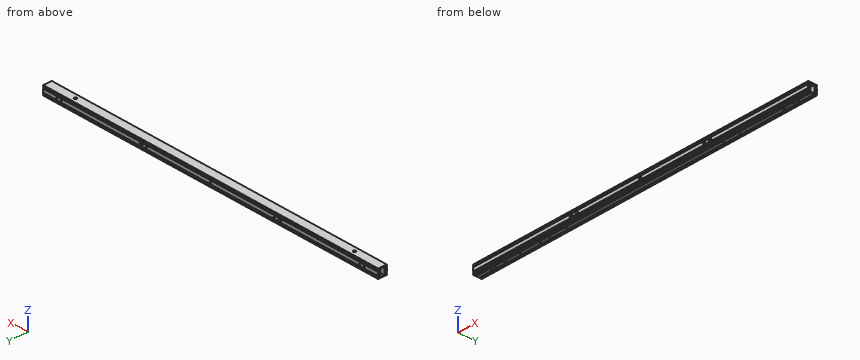
from build123d import *

# Parameters (mm, degrees)
SKETCH_1_W             = 23.5
SKETCH_1_H             = 12
EXTRUDE_1_DEPTH        = 601
HOLE_WIZARD_M6_1_D     = 5
HOLE_WIZARD_M6_1_DEPTH = 15
HOLE_WIZARD_M6_1_TIP   = 1.502151548
HOLE_WIZARD_M6_2_D     = 5
HOLE_WIZARD_M6_2_DEPTH = 15
HOLE_WIZARD_M6_2_TIP   = 1.502151548
SKETCH_8_R             = 4.5
CUT_EXTRUDE_1_DEPTH    = 602.935212461
HOLE_WIZARD_M6_3_D     = 5
HOLE_WIZARD_M6_3_DEPTH = 15
HOLE_WIZARD_M6_3_TIP   = 1.502151548
SKETCH_10_R            = 5.05
CUT_EXTRUDE_15_DEPTH   = 602.935212461
SKETCH_13_R            = 4.5
CUT_EXTRUDE_16_DEPTH   = 15
HOLE_WIZARD_M6_4_D     = 5
HOLE_WIZARD_M6_4_DEPTH = 15
HOLE_WIZARD_M6_4_TIP   = 1.502151548
HOLE_WIZARD_M6_5_D     = 5
HOLE_WIZARD_M6_5_DEPTH = 15
HOLE_WIZARD_M6_5_TIP   = 1.502151548


with BuildPart() as part:
    # 草图1 → 凸台-拉伸1 (new, symmetric)
    with BuildSketch(Plane(origin=(0, 0, 0), x_dir=(0, 0, -1), z_dir=(1, 0, 0))):
        with BuildLine():
            Line((-14, 15), (-11.5, 15))
            Line((-11.5, 15), (-11.5, 13.5))
            Line((-11.5, 13.5), (-11.4, 13.5))
            ThreePointArc((-11.4, 13.5), (-11.117157288, 13.382842712), (-11, 13.1))
            Line((-11, 13.1), (-11, 12))
            Line((-11, 12), (-9.5, 12))
            Line((-9.5, 12), (-9.5, 15))
            Line((-9.5, 15), (-8, 15))
            Line((-8, 15), (-8, 12.5))
            Line((-8, 12.5), (-5, 12.5))
            Line((-5, 12.5), (-5, 15))
            Line((-5, 15), (5, 15))
            Line((5, 15), (5, 12.5))
            Line((5, 12.5), (8, 12.5))
            Line((8, 12.5), (8, 15))
            Line((8, 15), (9.5, 15))
            Line((9.5, 15), (9.5, 12))
            Line((9.5, 12), (11, 12))
            Line((11, 12), (11, 13.1))
            ThreePointArc((11, 13.1), (11.117157288, 13.382842712), (11.4, 13.5))
            Line((11.4, 13.5), (11.5, 13.5))
            Line((11.5, 13.5), (11.5, 15))
            Line((11.5, 15), (14, 15))
            ThreePointArc((14, 15), (14.707106781, 14.707106781), (15, 14))
            Line((15, 14), (15, 8))
            Line((15, 8), (12.5, 8))
            Line((12.5, 8), (12.5, 5))
            Line((12.5, 5), (15, 5))
            Line((15, 5), (15, -5))
            Line((15, -5), (12.5, -5))
            Line((12.5, -5), (12.5, -8))
            Line((12.5, -8), (15, -8))
            Line((15, -8), (15, -14))
            ThreePointArc((15, -14), (14.707106781, -14.707106781), (14, -15))
            Line((14, -15), (11.5, -15))
            Line((11.5, -15), (11.5, -13.5))
            Line((11.5, -13.5), (11.4, -13.5))
            ThreePointArc((11.4, -13.5), (11.117157288, -13.382842712), (11, -13.1))
            Line((11, -13.1), (11, -12))
            Line((11, -12), (9.5, -12))
            Line((9.5, -12), (9.5, -15))
            Line((9.5, -15), (8, -15))
            Line((8, -15), (8, -12.5))
            Line((8, -12.5), (5, -12.5))
            Line((5, -12.5), (5, -15))
            Line((5, -15), (-5, -15))
            Line((-5, -15), (-5, -12.5))
            Line((-5, -12.5), (-8, -12.5))
            Line((-8, -12.5), (-8, -15))
            Line((-8, -15), (-9.5, -15))
            Line((-9.5, -15), (-9.5, -12))
            Line((-9.5, -12), (-11, -12))
            Line((-11, -12), (-11, -13.1))
            ThreePointArc((-11, -13.1), (-11.117157288, -13.382842712), (-11.4, -13.5))
            Line((-11.4, -13.5), (-11.5, -13.5))
            Line((-11.5, -13.5), (-11.5, -15))
            Line((-11.5, -15), (-14, -15))
            ThreePointArc((-14, -15), (-14.707106781, -14.707106781), (-15, -14))
            Line((-15, -14), (-15, 14))
            ThreePointArc((-15, 14), (-14.707106781, 14.707106781), (-14, 15))
        make_face()
        with BuildLine():
            Line((12, -10.5), (12, -8.5))
            ThreePointArc((12, -8.5), (11.853553391, -8.146446609), (11.5, -8))
            Line((11.5, -8), (-11.5, -8))
            ThreePointArc((-11.5, -8), (-11.853553391, -8.146446609), (-12, -8.5))
            Line((-12, -8.5), (-12, -10.5))
            ThreePointArc((-12, -10.5), (-11.853553391, -10.853553391), (-11.5, -11))
            Line((-11.5, -11), (11.5, -11))
            ThreePointArc((11.5, -11), (11.853553391, -10.853553391), (12, -10.5))
        make_face(mode=Mode.SUBTRACT)
        with BuildLine():
            Line((-11.5, 11), (11.5, 11))
            ThreePointArc((11.5, 11), (11.853553391, 10.853553391), (12, 10.5))
            Line((12, 10.5), (12, 8.5))
            ThreePointArc((12, 8.5), (11.853553391, 8.146446609), (11.5, 8))
            Line((11.5, 8), (-11.5, 8))
            ThreePointArc((-11.5, 8), (-11.853553391, 8.146446609), (-12, 8.5))
            Line((-12, 8.5), (-12, 10.5))
            ThreePointArc((-12, 10.5), (-11.853553391, 10.853553391), (-11.5, 11))
        make_face(mode=Mode.SUBTRACT)
        Rectangle(SKETCH_1_W, SKETCH_1_H, mode=Mode.SUBTRACT)
    extrude(amount=EXTRUDE_1_DEPTH, both=True)

    # M6 螺纹孔1
    with Locations(Plane(origin=(0, 0, -15), x_dir=(-1, 0, 0), z_dir=(0, 0, -1))):
        with Locations((-551, 0), (-536, 0), (536, 0), (551, 0)):
            Hole(HOLE_WIZARD_M6_1_D / 2, depth=HOLE_WIZARD_M6_1_DEPTH)
            with Locations((0, 0, -(HOLE_WIZARD_M6_1_DEPTH + HOLE_WIZARD_M6_1_TIP / 2))):  # 118° drill point
                Cone(0, HOLE_WIZARD_M6_1_D / 2, HOLE_WIZARD_M6_1_TIP, mode=Mode.SUBTRACT)

    # M6 螺纹孔2
    with Locations(Plane(origin=(0, 15, 0), x_dir=(-1, 0, 0), z_dir=(0, 1, 0))):
        with Locations((551, 0), (536, 0), (-536, 0), (-551, 0)):
            Hole(HOLE_WIZARD_M6_2_D / 2, depth=HOLE_WIZARD_M6_2_DEPTH)
            with Locations((0, 0, -(HOLE_WIZARD_M6_2_DEPTH + HOLE_WIZARD_M6_2_TIP / 2))):  # 118° drill point
                Cone(0, HOLE_WIZARD_M6_2_D / 2, HOLE_WIZARD_M6_2_TIP, mode=Mode.SUBTRACT)

    # 草图8 → 切除-拉伸1 (cut, through all)
    with BuildSketch(Plane.XY.offset(15)):
        with Locations((-501, 0)):
            Circle(SKETCH_8_R)
        with Locations((501, 0)):
            Circle(SKETCH_8_R)
    extrude(amount=-CUT_EXTRUDE_1_DEPTH, mode=Mode.SUBTRACT)

    # M6 螺纹孔3
    with Locations(Plane(origin=(0, 15, 0), x_dir=(-1, 0, 0), z_dir=(0, 1, 0))):
        with Locations((229, 0), (1, 0), (-229, 0)):
            Hole(HOLE_WIZARD_M6_3_D / 2, depth=HOLE_WIZARD_M6_3_DEPTH)
            with Locations((0, 0, -(HOLE_WIZARD_M6_3_DEPTH + HOLE_WIZARD_M6_3_TIP / 2))):  # 118° drill point
                Cone(0, HOLE_WIZARD_M6_3_D / 2, HOLE_WIZARD_M6_3_TIP, mode=Mode.SUBTRACT)

    # 草图10 → 切除-拉伸15 (cut, through all)
    with BuildSketch(Plane(origin=(0, 15, 0), x_dir=(-1, 0, 0), z_dir=(0, 1, 0))):
        with Locations(Location((249, 0, 0), (0, 0, 90))):
            Circle(SKETCH_10_R)
        with Locations(Location((-249, 0, 0), (0, 0, 90))):
            Circle(SKETCH_10_R)
    extrude(amount=-CUT_EXTRUDE_15_DEPTH, mode=Mode.SUBTRACT)

    # 草图13 → 切除-拉伸16 (cut)
    with BuildSketch(Plane.XZ.offset(15)):
        with Locations(Location((229, 0, 0), (0, 0, 90))):
            Circle(SKETCH_13_R)
        with Locations(Location((-1, 0, 0), (0, 0, 90))):
            Circle(SKETCH_13_R)
        with Locations(Location((-229, 0, 0), (0, 0, 90))):
            Circle(SKETCH_13_R)
    extrude(amount=-CUT_EXTRUDE_16_DEPTH, mode=Mode.SUBTRACT)

    # M6 螺纹孔4
    with Locations(Plane(origin=(0, 0, -15), x_dir=(-1, 0, 0), z_dir=(0, 0, -1))):
        with Locations((341, 0), (281, 0), (-281, 0), (-341, 0)):
            Hole(HOLE_WIZARD_M6_4_D / 2, depth=HOLE_WIZARD_M6_4_DEPTH)
            with Locations((0, 0, -(HOLE_WIZARD_M6_4_DEPTH + HOLE_WIZARD_M6_4_TIP / 2))):  # 118° drill point
                Cone(0, HOLE_WIZARD_M6_4_D / 2, HOLE_WIZARD_M6_4_TIP, mode=Mode.SUBTRACT)

    # M6 螺纹孔5
    with Locations(Plane(origin=(0, 0, -15), x_dir=(-1, 0, 0), z_dir=(0, 0, -1))):
        with Locations((446, 0), (376, 0)):
            Hole(HOLE_WIZARD_M6_5_D / 2, depth=HOLE_WIZARD_M6_5_DEPTH)
            with Locations((0, 0, -(HOLE_WIZARD_M6_5_DEPTH + HOLE_WIZARD_M6_5_TIP / 2))):  # 118° drill point
                Cone(0, HOLE_WIZARD_M6_5_D / 2, HOLE_WIZARD_M6_5_TIP, mode=Mode.SUBTRACT)


solid = part.part
Source: CAD feature listing. Evaluate the final solid. Frame: model axes, mm. Round coordinates to 2 decimals unless told otherwise and drop trailing zeros. Write item = value, one per line. Start each with the question number.
Item 1: First-contact query: pin 1 Ø6 at (x, z) = (-249, 0) entering from -Y; pin 2 Ø0.8 at (x, z) = (-68, 10.5) entering from +Y; pin 3 Ø6.5 at (x, z) = (229, 0) entering from -Y; pin 4 Ø1.5 at (x, y) = (-141.5, 6.5) entering from -Z. Flat tips, straight axial feed; report the tip coordinate or a pass-through.
Item 2: Section query A-A on x = 468. Count the separate pieces of the cut face and the enclosed holes in it, plus the area to 3 significant figures.
Item 3: Material intervals for line 1 (Y direction, x = -272, z = -7); line 2 (Y direction, x = -376, z = -14.2); line 3 (Z direction, x = 58, y = -12.75), sorted ascending.
Results list:
q1.pin_1 = through
q1.pin_2 = 12
q1.pin_3 = 6
q1.pin_4 = -12.5
q2.separate_pieces = 1
q2.enclosed_holes = 3
q2.area = 407 mm²
q3.line_1 = -12.5 to -11, -8 to -6, 6 to 8, 11 to 12.5
q3.line_2 = -14.98 to -8, -5 to -2.5, 2.5 to 5, 8 to 14.98
q3.line_3 = -15 to -11, -9.5 to -8, -5 to 5, 8 to 9.5, 11 to 15
